Could you check a few things on this drawing? It's one solid part, dimensions in mm from its lowest x, y, z. A direction names the side the tool comes from. Round coordinates to 2 decimals unless told otherwise and drop trailing zeros. Loops run counter-clockwise (first coordinate to the right, second up) from the corner with the lowest first, then second, coordinate; pieces in that order, holes last. Notation, with made-up numbers: M 9,53 L 18,53 A13 ccw 18,64 Z; hole C -38,-14.75 d3. An arc over 180 degrees is marked long. Answer as CSV lines item,"result".
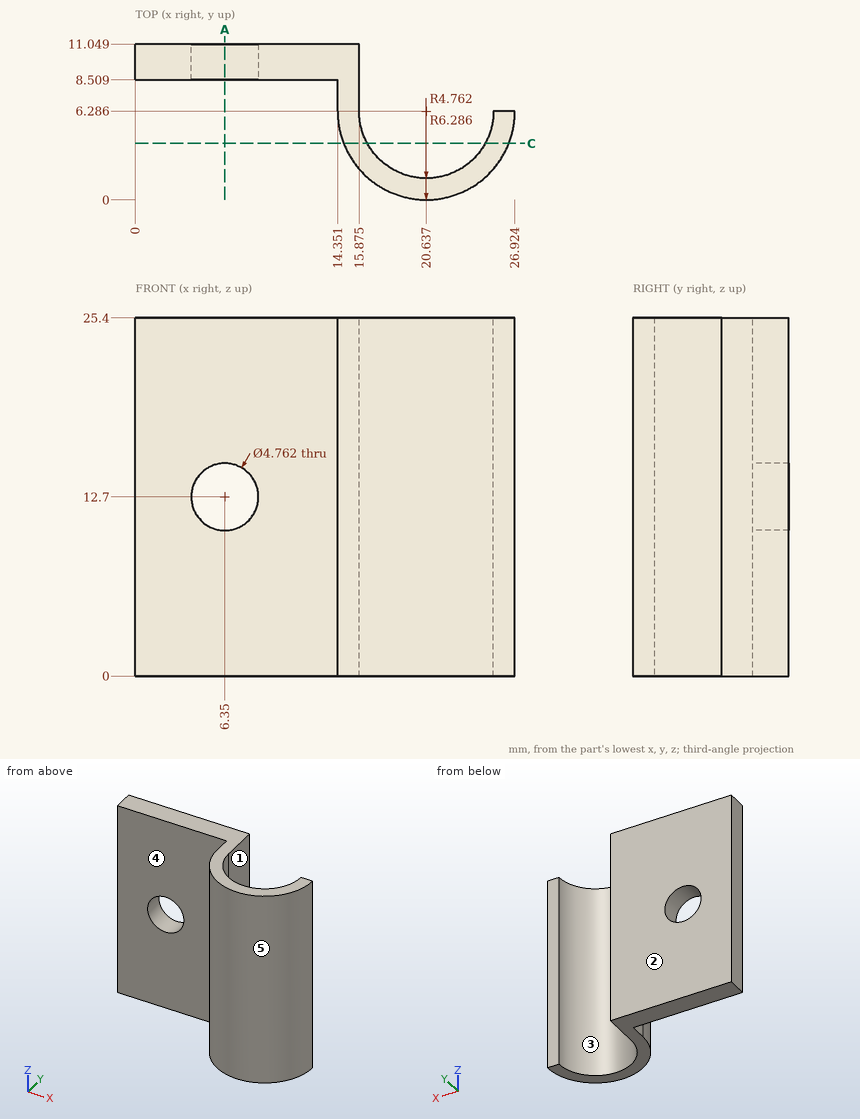
Item 1: If we section it at A-A on x = 6.35: Write out the boundary of the cut face in (y, z).
Output:
outline,"M 8.51,0 L 11.05,0 L 11.05,10.32 L 8.51,10.32 Z; M 8.51,15.08 L 11.05,15.08 L 11.05,25.4 L 8.51,25.4 Z"
Item 2: We'd pull the mould along X, two halves only. Please class the marked faces 3, 4 and 5: released by +X, released by -X, zero draft, split by the parting line, or undercut.
Output:
face 3,"undercut"
face 4,"zero draft"
face 5,"split by the parting line"
Item 3: Will these pins go through, and if not, where does the flat tip stop? pin 1 (12 mm diameter, centred on x = 22, z = 4, fed in from +Y); pin 2 (6 mm diameter, centred on y = 9, z = 3, fed in from -X); pin 3 (3 mm diameter, centred on x = 6, z = 21.5, fed in from -Y); pin 4 (1.4 mm diameter, centred on y = 9, z = 7, fed in from +X) (1 decimal).
Output:
pin 1,"stops at y = 6.29"
pin 2,"stops at x = 0"
pin 3,"stops at y = 8.51"
pin 4,"stops at x = 15.9"
Item 4: If I drill on line 1 along Z through (x, y) = (6.35, 10.3); line 2 along X through (y, z) = (10.35, 12.7) (1 decimal); line 3 along Y through (x, z) = (6, 3.75), over which ranges is the centre line in solid material (lowest first)? Write a range as from..to.
Output:
line 1,"z = 0..10.32, 15.08..25.4"
line 2,"x = 0..4, 8.7..15.9"
line 3,"y = 8.51..11.05"
Item 5: On a 3-axis mill with a long thin cutter (end or side, diameter ignored), from which of +Z, -Z, +X, -X, +Y, -Y can I reach the whole of each face in a straight line? I mean the marked faces 1 and 2. Say none if no direction works.
Output:
face 1,"+Z, -Z, +X, +Y"
face 2,"+Z, -Z, +X, -X, +Y"
Item 6: If we section it at C-C on y = 4: Write out the boundary of the cut face in (x, z) (1 decimal).
Output:
outline,"M 14.8,0 L 16.5,0 L 16.5,25.4 L 14.8,25.4 Z; M 24.8,0 L 26.5,0 L 26.5,25.4 L 24.8,25.4 Z"
